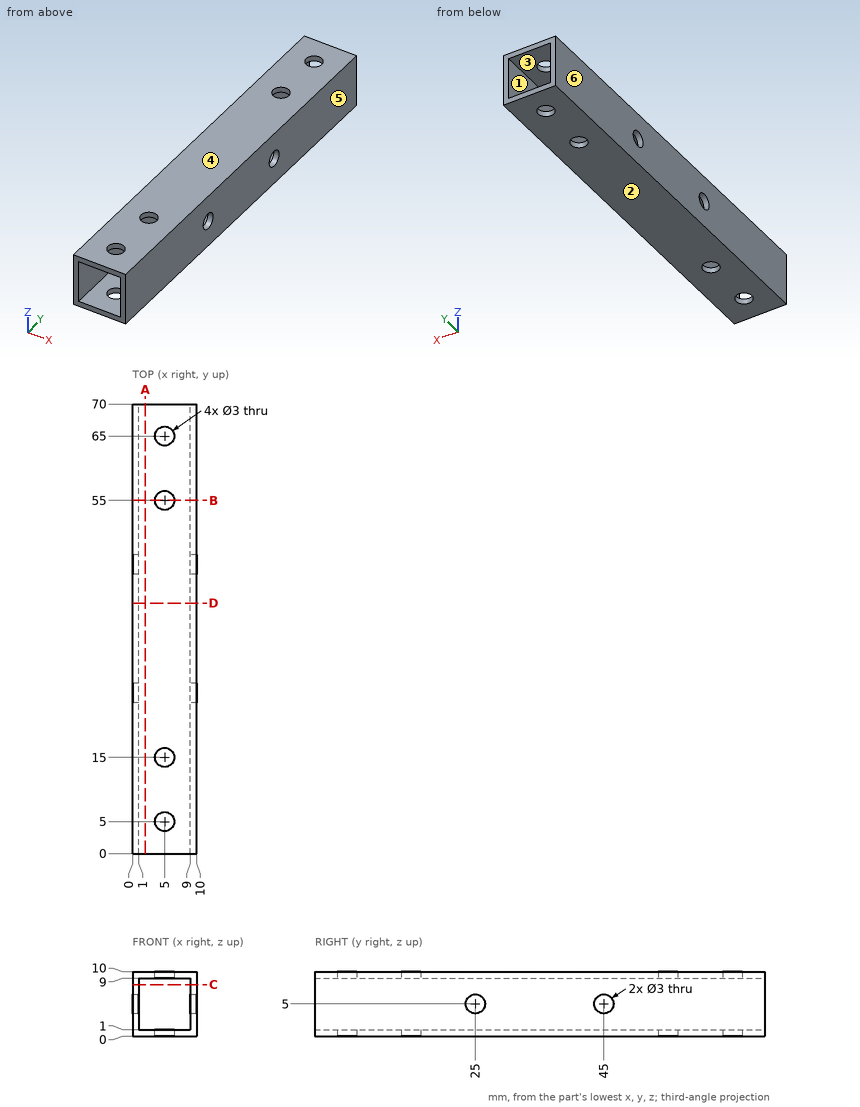
Source: three-view drawing plus pictorial views. Frame: mm from the lowest corner of the part. A direction names the side the tool comes from. Give positions to 0.01 mm unless a question says otherwise; leave off trailing zeros. Order: outer loops, then holes, each group sorted by start corner. A loop starts at its lowest first (then second) coordinate and runs counter-clockwise, first axis right, second up. Notation, with made-up numbers: (-6.75, -13.5) - (18.25, -13.5) arc R18 ccw to (18.25, -1.5) - close; hole circle Ø1 at (71, 47). An arc over 180 degrees is marked (long way). Answer as a JSON object with one key per item and string values. Group by question number.
Q1. Mould query, pull axis X, two halves, no side actions, for the marked faces 3, 4, 5 and 6. Classes: pulls with the +X half, pulls with the -X half, needs draft (parallel to the pull), parting line crosses it, or undercut.
Q2. Cut plane A-A, the plane x = 2. Output: boundary loops of the cut face in (y, z).
Q3. Cut plane C-C, the plane z = 8. Output: boundary loops of the cut face in (x, y).
Q4. First-contact query: pin 1 Ø2.5 at (x, y) = (5, 65) entering from +Z. Flat tip, straight axial feed; report the tip coordinate or a pass-through.
Q5. Set-up query: the marked faces 1 and 2. Return all of +Z, -Z, +X, -X, +Y, -Y with unobstructed straight access to the full face (end or side cutting, diameter ignored); none if empty.
Q6. Cut plane D-D, the plane y = 39. Output: boundary loops of the cut face in (x, z).
Q7. Line query: probe 1 along Y at (x, z) = (9.4, 5); probe 2 along Y at (x, z) = (5, 9.8); probe 3 along X at (y, z) = (61.5, 2). Output: solid intervals per line, ascending.
Q8. Cut plane B-B, the plane y = 55. Output: boundary loops of the cut face in (x, z).
Results:
{
 "1": {"face 3": "undercut", "face 4": "needs draft", "face 5": "pulls with the +X half", "face 6": "pulls with the -X half"},
 "2": {"outline": "(0, 0) - (70, 0) - (70, 1) - (0, 1) - close; (0, 9) - (70, 9) - (70, 10) - (0, 10) - close"},
 "3": {"outline": "(0, 0) - (1, 0) - (1, 70) - (0, 70) - close; (9, 0) - (10, 0) - (10, 70) - (9, 70) - close"},
 "4": {"pin 1": "through"},
 "5": {"face 1": "+Y, -Y", "face 2": "-Z, +X, -X, +Y, -Y"},
 "6": {"outline": "(0, 0) - (10, 0) - (10, 10) - (0, 10) - close; hole (1, 1) - (9, 1) - (9, 9) - (1, 9) - close"},
 "7": {"probe 1": "0 to 23.5, 26.5 to 43.5, 46.5 to 70", "probe 2": "0 to 3.5, 6.5 to 13.5, 16.5 to 53.5, 56.5 to 63.5, 66.5 to 70", "probe 3": "0 to 1, 9 to 10"},
 "8": {"outline": "(0, 0) - (3.5, 0) - (3.5, 1) - (1, 1) - (1, 9) - (3.5, 9) - (3.5, 10) - (0, 10) - close; (6.5, 0) - (10, 0) - (10, 10) - (6.5, 10) - (6.5, 9) - (9, 9) - (9, 1) - (6.5, 1) - close"}
}
